Design review of the part built by this model. Coordinates are the model's own, in mm. A direction names the side the tool comes from. Give positions to 0.01 mm unless a question says otherwise; leave off trailing zeros. Loops run counter-clockwise (first coordinate to the right, second up) from the corner with the lowest first, then second, coordinate; pieces in that order, holes last. Notation, with made-up numbers: (55, 27) -> (109, 27) arc R19 ccw to (109, 51) -> close; hole circle Ø3 at (-18, 67.5). An arc over 180 degrees is marked (long way). Answer in a Markdown table with one row per item. Add a question column.
(1) For pin 1 (6 mm diameter, centred on x = 3.5, y = 2.5, fed in from +Z); pin 2 (1 mm diameter, centred on y = 6.5, z = 0.5, fed in from +X); pin 3 (1.8 mm diameter, centred on x = 13.09, y = 12.71, fed in from +Z), all flat-tipped, find the tip position at first contact; note any pin that passes through.
(2) For line 1 (X direction, y = 3, z = 1.3); line 2 (Y direction, x = 6, z = 1.15); line 3 (X direction, y = 0.25, z = 0.75), list the stretches that pass through material, from the lowest coordinate up.
(3) Consider section D-D on y = 3.75. Write out the cut boundary in (x, z).
(4) For faces 1 (the cylindrical face through (1.134, -1.287, 1.38)), 2 (the flat face through (9, 10.713, 1)), list the 3-axis set-ups (+Z, -Z, +X, -X, +Y, -Y) from which the entire face can be reached by the end or side of a thin tool; tool diameter is ignored.
(5) Consider section C-C on x = 1.5. Write out the cut boundary in (y, z) (3 decimals), then the cut area to 3 significant figures.
(6) Draft analysis for pull direction Y (two halves, no side actions). For faces 3 (the cylindrical face through (12.09, 12.76, 1.38)), 4 (the flat face through (6, 14.713, 1)), 5 (the flat face through (3.09, 5, 1)), state which applies: +Y half, -Y half, draft (parallel to the pull), parting line (faces both ways), or undercut.
(7) Consider section A-A on x = 13.5. Write out the cut boundary in (y, z) (3 decimals).
(8) Consider section B-B on z = 2.4. Write out the cut boundary in (x, y).
from build123d import *

# Parameters (mm, degrees)
SKETCH1_R           = 1
BOSS_EXTRUDE2_DEPTH = 2.8
FILLET1_R           = 1


with BuildPart() as part:
    # Sketch1 → Boss-Extrude2 (new body)
    with BuildSketch(Plane.XY):
        with BuildLine():
            Line((-0.910186913, 0.71299639), (-0.910186913, 14.71299639))
            Line((-0.910186913, 14.71299639), (13.089813087, 14.71299639))
            ThreePointArc((13.089813087, 14.71299639), (15.089813087, 12.71299639), (13.089813087, 10.71299639))
            Line((13.089813087, 10.71299639), (3.089813087, 10.71299639))
            Line((3.089813087, 10.71299639), (3.089813087, 0.71299639))
            ThreePointArc((3.089813087, 0.71299639), (1.089813087, -1.28700361), (-0.910186913, 0.71299639))
        make_face()
        with Locations((1.089813087, 0.71299639)):
            Circle(SKETCH1_R, mode=Mode.SUBTRACT)
        with Locations((13.089813087, 12.71299639)):
            Circle(SKETCH1_R, mode=Mode.SUBTRACT)
    extrude(amount=BOSS_EXTRUDE2_DEPTH)

    # Fillet1
    fillet1_edges = [part.edges().sort_by_distance(p)[0] for p in [
        (3.089813087, 10.71299639, 1.4),
        (-0.910186913, 14.71299639, 1.4),
    ]]
    fillet(fillet1_edges, radius=FILLET1_R)


solid = part.part
Values follow:
| question | item | result |
|---|---|---|
| 1 | pin 1 | z = 2.8 |
| 1 | pin 2 | x = 3.09 |
| 1 | pin 3 | through |
| 2 | line 1 | -0.91 to 3.09 |
| 2 | line 2 | 10.71 to 14.71 |
| 2 | line 3 | -0.86 to 0.2, 1.98 to 3.04 |
| 3 | outline | (-0.91, 0) -> (3.09, 0) -> (3.09, 2.8) -> (-0.91, 2.8) -> close |
| 4 | face 1 | +Z, -Z, -Y |
| 4 | face 2 | +Z, -Z, +X, -Y |
| 5 | outline | (-1.244, 0) -> (-0.199, 0) -> (-0.199, 2.8) -> (-1.244, 2.8) -> close; (1.625, 0) -> (14.713, 0) -> (14.713, 2.8) -> (1.625, 2.8) -> close |
| 5 | area | 39.6 mm2 |
| 6 | face 3 | undercut |
| 6 | face 4 | +Y half |
| 6 | face 5 | draft |
| 7 | outline | (10.756, 0) -> (11.801, 0) -> (11.801, 2.8) -> (10.756, 2.8) -> close; (13.625, 0) -> (14.67, 0) -> (14.67, 2.8) -> (13.625, 2.8) -> close |
| 8 | outline | (-0.91, 0.71) arc R2 ccw to (3.09, 0.71) -> (3.09, 9.71) arc R1 cw to (4.09, 10.71) -> (13.09, 10.71) arc R2 ccw to (13.09, 14.71) -> (0.09, 14.71) arc R1 ccw to (-0.91, 13.71) -> close; hole circle Ø2 at (1.09, 0.71); hole circle Ø2 at (13.09, 12.71) |
